```python
from build123d import *

# Parameters (mm, degrees)
BOSS_EXTRUDE1_DEPTH = 75


with BuildPart() as part:
    # Sketch1 → Boss-Extrude1 (new, symmetric)
    with BuildSketch(Plane.XY):
        with BuildLine():
            ThreePointArc((-0.917765177, -38.883932695), (10.262933143, -17.63377253), (34.256460841, -18.576083835))
            ThreePointArc((34.256460841, -18.576083835), (69.499988538, -0.032823555), (34.256460841, 18.510436725))
            ThreePointArc((34.256460841, 18.510436725), (10.262933143, 17.568125421), (-0.917765177, 38.818285585))
            ThreePointArc((-0.917765177, 38.818285585), (-34.598463498, 60.06844575), (-33.035634121, 20.275025305))
            ThreePointArc((-33.035634121, 20.275025305), (-20.222804743, -0.032823555), (-33.035634121, -20.340672415))
            ThreePointArc((-33.035634121, -20.340672415), (-34.598463498, -60.13409286), (-0.917765177, -38.883932695))
        make_face()
        with BuildLine():
            Line((1.907111414, -11.957316484), (1.245826983, -9.922092276))
            ThreePointArc((1.245826983, -9.922092276), (-2.974669232, -9.547321245), (-6.661121842, -7.458515657))
            Line((-6.661121842, -7.458515657), (-8.330592399, -8.671457016))
            Line((-8.330592399, -8.671457016), (-10.681733408, -5.435389039))
            Line((-10.681733408, -5.435389039), (-9.051488804, -4.250947003))
            ThreePointArc((-9.051488804, -4.250947003), (-9.99981681, -0.060529116), (-9.102285822, 4.141061797))
            Line((-9.102285822, 4.141061797), (-10.720319811, 5.316632302))
            Line((-10.720319811, 5.316632302), (-8.369178802, 8.552700279))
            Line((-8.369178802, 8.552700279), (-6.751144813, 7.377129775))
            ThreePointArc((-6.751144813, 7.377129775), (-3.054553816, 9.522063904), (1.199967545, 9.92774284))
            Line((1.199967545, 9.92774284), (1.844677303, 11.911955447))
            Line((1.844677303, 11.911955447), (5.648903368, 10.67588747))
            Line((5.648903368, 10.67588747), (4.994934057, 8.663176887))
            ThreePointArc((4.994934057, 8.663176887), (8.112145375, 5.847486418), (9.797958971, 2))
            Line((9.797958971, 2), (12, 2))
            Line((12, 2), (12, -2))
            Line((12, -2), (9.797958971, -2))
            ThreePointArc((9.797958971, -2), (8.125687266, -5.828653915), (5.035070067, -8.639911424))
            Line((5.035070067, -8.639911424), (5.71133748, -10.721248507))
            Line((5.71133748, -10.721248507), (1.907111414, -11.957316484))
        make_face(mode=Mode.SUBTRACT)
    extrude(amount=BOSS_EXTRUDE1_DEPTH, both=True)


solid = part.part
```
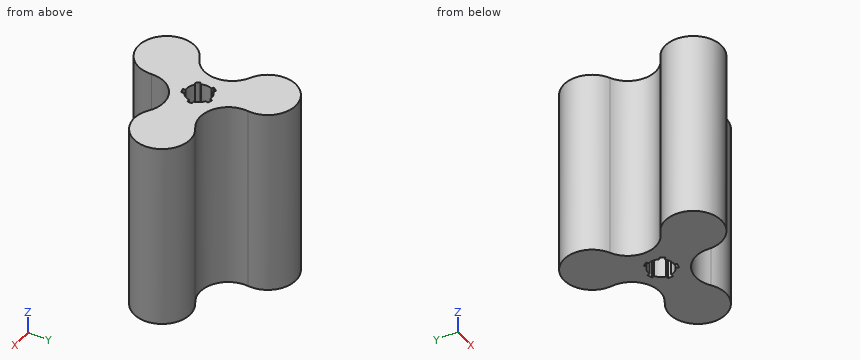
The model under review builds one solid part; all positions refer to its coordinate system, in mm. Coordinates: 2 decimals unless noted, no trailing zeros. Order: outer loops, then holes, each group sorted by start corner. A loop starts at its lowest first (then second) coordinate and runs counter-clockwise, first axis right, second up. Notation, with made-up numbers: (56.25, 50.25) -> (96.25, 50.25) arc R26 ccw to (96.25, 88.25) -> close; hole circle Ø5 at (40, 41). An arc over 180 degrees is marked (long way). Answer in a Markdown table with one row per item. Add a question column.
Item 1: We need section D-D on x = 60. Write out the cut boundary in (y, z), plus the area to 3 significant figures.
Item 2: Clearance check with flat-ended pins moving along their axes: pin 1 (1.8 mm diameter, centred on x = 10.5, z = 15, fed in from +Y); pin 2 (8 mm diameter, centred on x = 18, z = 13, fed in from -Y); pin 3 (8 mm diameter, centred on x = -16.5, z = -51.5, fed in from -Y). State where each tip first meets the part, or that it passes through.
Item 3: We need section B-B on z = 4. Write out the cut boundary in (x, y).
Item 4: We need section C-C on y = -30. Write out the cut boundary in (x, z), plus the area to 3 significant figures.
Item 5: We need section A-A on x = -23. Write out the cut boundary in (y, z), plus the area to 3 significant figures.
Item 6: To check wall thickness, follow probe 1 along Y at (x, z) = (6, -54.5); probe 2 along Y at (x, z) = (-32, 42); probe 3 along Y at (x, z) = (21, 18). State the ranges of each line that lie inside material, in increasing order.
Final values:
| question | item | result |
|---|---|---|
| 1 | outline | (-18.4, -75) -> (18.33, -75) -> (18.33, 75) -> (-18.4, 75) -> close |
| 1 | area | 5,510 mm2 |
| 2 | pin 1 | stops at y = 17.97 |
| 2 | pin 2 | stops at y = -15.91 |
| 2 | pin 3 | stops at y = -62.97 |
| 3 | outline | (-33.04, -20.34) arc R22.5 ccw (long way) to (-0.92, -38.88) arc R22.5 cw to (34.26, -18.58) arc R22.5 ccw (long way) to (34.26, 18.51) arc R22.5 cw to (-0.92, 38.82) arc R22.5 ccw (long way) to (-33.04, 20.28) arc R22.5 cw to start; hole (-10.72, 5.32) -> (-9.1, 4.14) arc R10 ccw to (-9.05, -4.25) -> (-10.68, -5.44) -> (-8.33, -8.67) -> (-6.66, -7.46) arc R10 ccw to (1.25, -9.92) -> (1.91, -11.96) -> (5.71, -10.72) -> (5.04, -8.64) arc R10 ccw to (9.8, -2) -> (12, -2) -> (12, 2) -> (9.8, 2) arc R10 ccw to (4.99, 8.66) -> (5.65, 10.68) -> (1.84, 11.91) -> (1.2, 9.93) arc R10 ccw to (-6.75, 7.38) -> (-8.37, 8.55) -> close |
| 4 | outline | (-43.17, -75) -> (0.17, -75) -> (0.17, 75) -> (-43.17, 75) -> close |
| 4 | area | 6,500 mm2 |
| 5 | outline | (-63.15, -75) -> (-10.86, -75) -> (-10.86, 75) -> (-63.15, 75) -> close; (10.8, -75) -> (63.08, -75) -> (63.08, 75) -> (10.8, 75) -> close |
| 5 | area | 15,700 mm2 |
| 6 | probe 1 | y = -20.82 to -8, 8 to 20.76 |
| 6 | probe 2 | y = -61.42 to -19.81, 19.75 to 61.35 |
| 6 | probe 3 | y = -14.63 to 14.56 |
